Geometry: final body of the model. Coordinates: model frame, mm. A direction names the side the tool comes from. Give positions to 0.01 mm unless a question says otherwise; leave off trailing zeros. Loops run counter-clockwise (first coordinate to the right, second up) from the corner with the lowest first, then second, coordinate; pieces in that order, holes last.
from build123d import *

# Parameters (mm, degrees)
BOSS_EXTRUDE1_DEPTH      = 20
BOSS_EXTRUDE1_DEPTH_BACK = 15
BOSS_EXTRUDE2_START      = -20
SKETCH1_3_R              = 1.75
BOSS_EXTRUDE2_DEPTH      = 5
CHAMFER1_SIZE            = 15
CHAMFER1_SIZE2           = 4.019237886
FILLET1_R                = 2


with BuildPart() as part:
    # Sketch1 → Boss-Extrude1 (new, two sides: drawn at the far end of the back side and taken through both)
    with BuildSketch(Plane.XY.offset(-BOSS_EXTRUDE1_DEPTH_BACK)):
        with BuildLine():
            ThreePointArc((-73.461980247, -100.14832099), (-102.624010348, -59.25), (-123.461980247, -13.545780611))
            Line((-123.461980247, -13.545780611), (-140.782488323, -23.545780611))
            Line((-140.782488323, -23.545780611), (-90.782488323, -110.14832099))
            Line((-90.782488323, -110.14832099), (-73.461980247, -100.14832099))
        make_face()
    extrude(amount=BOSS_EXTRUDE1_DEPTH + BOSS_EXTRUDE1_DEPTH_BACK)

    # Sketch1<3> → Boss-Extrude2 (add)
    # profile 1 of 2: a face of its own
    with BuildSketch(Plane.XY.offset(BOSS_EXTRUDE2_START)):
        with BuildLine():
            ThreePointArc((-73.461980247, -100.14832099), (-102.624010348, -59.25), (-123.461980247, -13.545780611))
            Line((-123.461980247, -13.545780611), (-140.782488323, -23.545780611))
            Line((-140.782488323, -23.545780611), (-90.782488323, -110.14832099))
            Line((-90.782488323, -110.14832099), (-73.461980247, -100.14832099))
        make_face()
    # profile 2 of 2: a face of its own
    with BuildSketch(Plane.XY.offset(BOSS_EXTRUDE2_START)):
        with BuildLine():
            Line((-114.801726209, -8.545780611), (-123.461980247, -13.545780611))
            ThreePointArc((-123.461980247, -13.545780611), (-102.624010348, -59.25), (-73.461980247, -100.14832099))
            Line((-73.461980247, -100.14832099), (-64.801726209, -95.14832099))
            Line((-64.801726209, -95.14832099), (-114.801726209, -8.545780611))
        make_face()
        with Locations(Location((-71.631853228, -93.318193971, 0), (0, 0, 180))):
            Circle(SKETCH1_3_R, mode=Mode.SUBTRACT)
        with Locations(Location((-116.631853228, -15.37590763, 0), (0, 0, 180))):
            Circle(SKETCH1_3_R, mode=Mode.SUBTRACT)
    extrude(amount=BOSS_EXTRUDE2_DEPTH)

    # Chamfer1
    chamfer1_edges = [part.edges().sort_by_distance(p)[0] for p in [
        (-115.782488323, -66.847050801, 20),
    ]]
    chamfer1_side = [part.faces().sort_by_distance(p)[0] for p in [
        (-115.782488323, -66.847050801, 0),
    ]]
    chamfer(chamfer1_edges, length=CHAMFER1_SIZE, length2=CHAMFER1_SIZE2, reference=chamfer1_side[0])

    # Fillet1
    fillet1_edges = [part.edges().sort_by_distance(p)[0] for p in [
        (-89.042107266, -109.143511518, 12.5),
        (-139.042107266, -22.54097114, 12.5),
    ]]
    fillet(fillet1_edges, radius=FILLET1_R)


solid = part.part
Item 1: Section query D-D on z = -5.5. Return loops of the section in (x, y), plus the area to 3 significant figures.
Values follow:
outline: (-140.78, -23.55) - (-90.78, -110.15) - (-73.46, -100.15) arc R262.5 cw to (-123.46, -13.55) - close
area: 1,680 mm2
Item 2: Section query B-B on x = -99.5. Return loops of the section in (y, z), plus the area to 3 significant figures.
Values follow:
outline: (-95.05, -20) - (-35.05, -20) - (-35.05, -15) - (-64.52, -15) - (-64.52, 20) - (-87.01, 20) - (-95.05, 5) - close
area: 1,310 mm2
Item 3: Draft query along X for faces 1 (the face through (-138.407, -22.833, 11.683)), 2 (the face through (-73.301, -93.844, -17.535)), 3 (the face through (-103, -59, -20)). Return one class per face: +X half, -X half, draft (parallel to the pull), parting line (faces both ways), or undercut.
Values follow:
face 1: -X half
face 2: undercut
face 3: draft
Item 4: Ray query, probe 1 along Z at (x, y) = (-79.5, -91); probe 2 along Y at (x, z) = (-116, -18); probe 3 along Y at (x, z) = (-134.5, 17). Return the intervals inside material, ascending.
Values follow:
probe 1: z = -20 to -15
probe 2: y = -66.47 to -17.01, -13.74 to -9.24
probe 3: y = -28 to -19.92
Item 5: Pin query (flat end, axial travel): pin 1 (2 mm diameter, centred on x = -76, z = -7.5, fed in from +Y); pin 2 (2 mm diameter, centred on x = -71.63, y = -93.32, fed in from -Z); pin 3 (10 mm diameter, centred on x = -91.5, z = -3, fed in from +Y); pin 4 (2 mm diameter, centred on x = -85.5, z = 0.5, fed in from +Y). Return the tip coordinate at first contact, or that it passes through.
Values follow:
pin 1: stops at y = -95.99
pin 2: passes through
pin 3: stops at y = -69.33
pin 4: stops at y = -83.88
Item 6: Section query C-C on z = -16.5. Return loops of the section in (x, y), plus the area to 3 significant figures.
Values follow:
outline: (-140.78, -23.55) - (-90.78, -110.15) - (-64.8, -95.15) - (-114.8, -8.55) - close; hole circle Ø3.5 at (-116.63, -15.38); hole circle Ø3.5 at (-71.63, -93.32)
area: 2,980 mm2
Item 7: Set-up query: faces 4 (the face through (-102.27, -59.86, 2.25)), 5 (the face through (-118.3, -15.9, -17.5)). Return all of +Z, -Z, +X, -X, +Y, -Y with unobstructed straight access to the full face (end or side cutting, diameter ignored); none if empty.
Values follow:
face 4: +Z, +X, +Y
face 5: +Z, -Z
Item 8: Section query A-A on y = -88. Return loops of the section in (x, z), plus the area to 3 significant figures.
Values follow:
outline: (-103.57, -20) - (-68.93, -20) - (-68.93, -15) - (-83.39, -15) - (-83.39, 20) - (-98.93, 20) - (-103.57, 5) - close
area: 845 mm2
